Geometry check sheet. Reference: the model listing, model coordinates, mm. Face numbers are marked on the shaded views. A direction names the side the tool comes from. Round coordinates to 2 decimals unless told otherwise and drop trailing zeros. Loops run counter-clockwise (first coordinate to the right, second up) from the corner with the lowest first, then second, coordinate; pieces in that order, holes last. Notation, with made-up numbers: M 3,-20.5 L 52,-20.5 A21 ccw 52,-10.5 Z; hole C -13.5,56.5 d7. An arc over 180 degrees is marked long. Use one line per item in the form item = value. Start each with the question number.
1. Draft check along Y on the marked faces 6, 7 and 8. Enter one of: pulls with the +Y half, pulls with the -Y half, needs draft (parallel to the pull), parting line crosses it, or undercut.
2. Set-up check for the marked faces 1, 2, 3, 4 and 5: record each of +Z, -Z, +X, -X, +Y, -Y from which the full face is reachable in a straight line by a thin tool's end or side.
3. Cross-section at A-A (x = -70). State how many separate pieces and enclosed holes the cut face has, then the cut area to 3 significant figures.
4. Material ranges on line 1 (Y direction, x = -46, z = 3); line 2 (X direction, y = -51.5, z = 12.25); line 3 (Y direction, x = 70, z = 7.75), recorded low to high.
5. Cross-section at B-B (z = -3). Record the boundary of the cut face in (x, y).
6. Go/stop test with flat-tipped pins: pin 1 (7 mm diameter, centred on x = 46, y = -51, fed in from -Z); pin 2 (12 mm diameter, centred on y = -34, z = 10.5, fed in from +X); pin 3 (1 mm diameter, centred on x = 17.5, z = -3, fed in from -Y); pin 4 (6 mm diameter, centred on x = 70, y = -69, fed in from +Z). Record where each tip stops, or that it passes through.
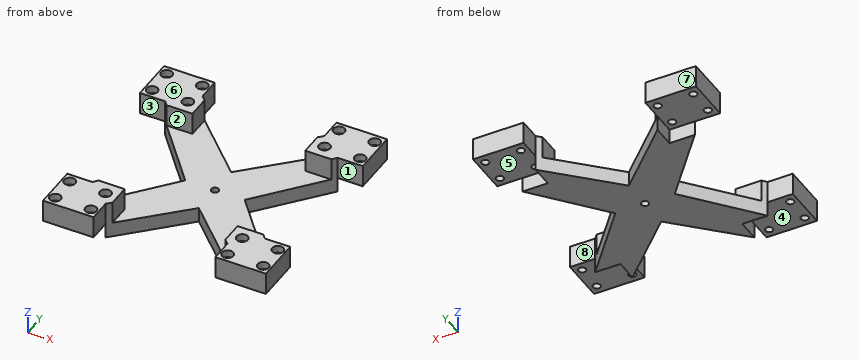
```python
from build123d import *

# Parameters (mm, degrees)
SKETCH1_W           = 150
SKETCH1_H           = 150
BOSS_EXTRUDE1_DEPTH = 15
CUT_EXTRUDE1_DEPTH  = 15
BOSS_EXTRUDE2_DEPTH = 25
CUT_EXTRUDE2_DEPTH  = 15
SKETCH5_R           = 2.5
CUT_EXTRUDE3_DEPTH  = 15
SKETCH7_R           = 2.5
CUT_EXTRUDE4_DEPTH  = 15
SKETCH8_R           = 3.8
CUT_EXTRUDE5_DEPTH  = 5
SKETCH10_R          = 2.5
CUT_EXTRUDE6_DEPTH  = 26
SKETCH11_R          = 3.8
CUT_EXTRUDE7_DEPTH  = 5
SKETCH12_R          = 2.5
CUT_EXTRUDE8_DEPTH  = 26
SKETCH13_R          = 3.8
CUT_EXTRUDE9_DEPTH  = 5
SKETCH14_R          = 2.5
CUT_EXTRUDE10_DEPTH = 26
SKETCH15_R          = 3.8
CUT_EXTRUDE11_DEPTH = 5


with BuildPart() as part:
    # Sketch1 → Boss-Extrude1 (new body)
    with BuildSketch(Plane.XY):
        Rectangle(SKETCH1_W, SKETCH1_H)
    extrude(amount=BOSS_EXTRUDE1_DEPTH)

    # Sketch2 → Cut-Extrude1 (cut)
    with BuildSketch(Plane.XY.offset(15)):
        Polygon((-41, 75), (-41, 60), (0, 20), (41, 60), (41, 75), align=None)
        Polygon((-20, 0), (-58, 45), (-75, 45), (-75, -45), (-58, -45), align=None)
        Polygon((58, 45), (20, 0), (58, -45), (75, -45), (75, 45), align=None)
        Polygon((41, -60), (0, -20), (-41, -60), (-41, -75), (41, -75), align=None)
    extrude(amount=-CUT_EXTRUDE1_DEPTH, mode=Mode.SUBTRACT)

    # Sketch3 → Boss-Extrude2 (add)
    with BuildSketch(Plane.XY.offset(15)):
        Polygon((-41, 45.069428085), (-58, 45.069428085), (-20, 0), (-58, -45), (-41, -45), (-41, -60), (0, -20), (41, -60), (41, -45), (58, -45), (20, 0), (58, 45), (41, 45), (41, 60), (0, 20), (-41, 60), align=None)
    extrude(amount=-BOSS_EXTRUDE2_DEPTH)

    # Sketch4 → Cut-Extrude2 (cut)
    with BuildSketch(Plane.XY.offset(15)):
        Polygon((-38, -42), (-38, -57.073170732), (0, -20), (38, -57.073170732), (38, -42), (55.466666667, -42), (20, 0), (55.466666667, 42), (37.925, 42), (37.925, 57), (0, 20), (-37.220661316, 56.312840308), (-37.426275475, 56.513439488), (-38, 57.073170732), (-38, 42), (-55.466666667, 42), (-20, 0), (-55.466666667, -42), align=None)
    extrude(amount=-CUT_EXTRUDE2_DEPTH, mode=Mode.SUBTRACT)

    # Sketch5 → Cut-Extrude3 (cut)
    with BuildSketch(Plane.XY):
        Circle(SKETCH5_R)
    extrude(amount=-CUT_EXTRUDE3_DEPTH, mode=Mode.SUBTRACT)

    # Sketch7 → Cut-Extrude4 (cut)
    with BuildSketch(Plane.XY.offset(15)):
        with Locations((70, -51)):
            Circle(SKETCH7_R)
        with Locations((46, -51)):
            Circle(SKETCH7_R)
        with Locations((46, -69)):
            Circle(SKETCH7_R)
        with Locations((70, -69)):
            Circle(SKETCH7_R)
    extrude(amount=-CUT_EXTRUDE4_DEPTH, mode=Mode.SUBTRACT)

    # Sketch8 → Cut-Extrude5 (cut)
    with BuildSketch(Plane.XY.offset(15)):
        with Locations((46, -51)):
            Circle(SKETCH8_R)
        with Locations((70, -51)):
            Circle(SKETCH8_R)
        with Locations((70, -69)):
            Circle(SKETCH8_R)
        with Locations((46, -69)):
            Circle(SKETCH8_R)
    extrude(amount=-CUT_EXTRUDE5_DEPTH, mode=Mode.SUBTRACT)

    # Sketch10 → Cut-Extrude6 (cut, through all)
    with BuildSketch(Plane.XY.offset(15)):
        with Locations((-46, -69)):
            Circle(SKETCH10_R)
        with Locations((-46, -51)):
            Circle(SKETCH10_R)
        with Locations((-70, -51)):
            Circle(SKETCH10_R)
        with Locations((-70, -69)):
            Circle(SKETCH10_R)
    extrude(amount=-CUT_EXTRUDE6_DEPTH, mode=Mode.SUBTRACT)

    # Sketch11 → Cut-Extrude7 (cut)
    with BuildSketch(Plane.XY.offset(15)):
        with Locations((-70, -51)):
            Circle(SKETCH11_R)
        with Locations((-46, -51)):
            Circle(SKETCH11_R)
        with Locations((-70, -69)):
            Circle(SKETCH11_R)
        with Locations((-46, -69)):
            Circle(SKETCH11_R)
    extrude(amount=-CUT_EXTRUDE7_DEPTH, mode=Mode.SUBTRACT)

    # Sketch12 → Cut-Extrude8 (cut, through all)
    with BuildSketch(Plane.XY.offset(15)):
        with Locations((46, 69)):
            Circle(SKETCH12_R)
        with Locations((70, 69)):
            Circle(SKETCH12_R)
        with Locations((70, 51)):
            Circle(SKETCH12_R)
        with Locations((46, 51)):
            Circle(SKETCH12_R)
    extrude(amount=-CUT_EXTRUDE8_DEPTH, mode=Mode.SUBTRACT)

    # Sketch13 → Cut-Extrude9 (cut)
    with BuildSketch(Plane.XY.offset(15)):
        with Locations((70, 69)):
            Circle(SKETCH13_R)
        with Locations((46, 69)):
            Circle(SKETCH13_R)
        with Locations((46, 51)):
            Circle(SKETCH13_R)
        with Locations((70, 51)):
            Circle(SKETCH13_R)
    extrude(amount=-CUT_EXTRUDE9_DEPTH, mode=Mode.SUBTRACT)

    # Sketch14 → Cut-Extrude10 (cut, through all)
    with BuildSketch(Plane.XY.offset(15)):
        with Locations((-70, 69)):
            Circle(SKETCH14_R)
        with Locations((-46, 69)):
            Circle(SKETCH14_R)
        with Locations((-46, 51)):
            Circle(SKETCH14_R)
        with Locations((-70, 51)):
            Circle(SKETCH14_R)
    extrude(amount=-CUT_EXTRUDE10_DEPTH, mode=Mode.SUBTRACT)

    # Sketch15 → Cut-Extrude11 (cut)
    with BuildSketch(Plane.XY.offset(15)):
        with Locations((-70, 69)):
            Circle(SKETCH15_R)
        with Locations((-46, 69)):
            Circle(SKETCH15_R)
        with Locations((-46, 51)):
            Circle(SKETCH15_R)
        with Locations((-70, 51)):
            Circle(SKETCH15_R)
    extrude(amount=-CUT_EXTRUDE11_DEPTH, mode=Mode.SUBTRACT)


solid = part.part
```
Reported:
q1.face_6 = needs draft
q1.face_7 = pulls with the +Y half
q1.face_8 = undercut
q2.face_1 = +Z, -Z, +X
q2.face_2 = +Z, +X, -X
q2.face_3 = +Z, -Z, -X
q2.face_4 = -Z, -X, -Y
q2.face_5 = -Z, +X, +Y
q3.separate_pieces = 6
q3.enclosed_holes = 0
q3.area = 548 mm²
q4.line_1 = -75 to -71.5, -66.5 to -53.5, -48.5 to -42, 42 to 48.5, 53.5 to 66.5, 71.5 to 75
q4.line_2 = -75 to -73.77, -66.23 to -49.77, -42.23 to -38, 38 to 42.23, 49.77 to 66.23, 73.77 to 75
q4.line_3 = -75 to -71.5, -66.5 to -53.5, -48.5 to -45, 45 to 48.5, 53.5 to 66.5, 71.5 to 75
q5.outline = M -58,-45 L -41,-45 L -41,-60 L 0,-20 L 41,-60 L 41,-45 L 58,-45 L 20,0 L 58,45 L 41,45 L 41,60 L 0,20 L -41,60 L -41,45.07 L -58,45.07 L -20,0 Z; hole C 0,0 d5
q6.pin_1 = 0
q6.pin_2 = through
q6.pin_3 = -37.56
q6.pin_4 = 10
